CAD build for the part. Positions are in the model's coordinates, mm. Face numbers are marked on the shaded views. Coordinates: 2 decimals unless noted, no trailing zeros. Write each loop counter-clockwise with the first axis right and the second up, starting at its lowest first coordinate (ties: lowest second). Pieces come first, ordered by that corner, then holes. Notation, with made-up numbers: (64.5, -26.75) - (80.5, -26.75) arc R18 cw to (80.5, -7.75) - close; hole circle Ø6 at (-25, 65). An arc over 180 degrees is marked (long way). Answer in a Markdown table with one row per item. Add a question column.
Q1. Band-saw the part on D-D (y = 14). List the corners of the cut face in (x, z).
Q2. Two-plate mould, pull along X, no slides. Class the marked faces 1, 2, 3 and 4: +X half, -X half, draft (parallel to the pull), parting line (faces both ways), or undercut.
Q3. Drill centre lines: line 1 along Y through (x, z) = (-10, -0.25); line 2 along Y through (x, z) = (-13, 2); line 3 along X through (y, z) = (52, 0.4). Where is each one in solid material? Low to high. Write a range as from..to.
Q4. Band-saw the part on B-B (x = -10). List the corners of the cut face in (y, z), and give its area (3 significant figures).
Q5. Band-saw the part on A-A (y = 58). List the corners of the cut face in (x, z).
Q6. Band-saw the part on C-C (z = -0.8). List the corners of the cut face in (x, y), and give its area (3 significant figures).
Autodesk Inventor part; units mm, degrees
ref_plane "YZ Plane" through (0, 0, 0) normal (1, 0, 0) x (0, 1, 0)
ref_plane "XZ Plane" through (0, 0, 0) normal (0, 1, 0) x (-1, 0, 0)
ref_plane "XY Plane" through (0, 0, 0) normal (0, 0, 1) x (1, 0, 0)
sketch "Sketch1" plane through (0, 0, 0) normal (0, 0, 1) x (1, 0, 0)
  line L0 (-5, 0) -> (-15, 0)
  line L1 (-20, 5) -> (-20, 60)
  line L2 (-15, 65) -> (-5, 65)
  line L3 (0, 60) -> (0, 5)
  circle A0 centre (-10, 55) radius 5
  circle A1 centre (-10, 10) radius 5
  arc A2 (-15, 65) -> (-20, 60) centre (-15, 60) ccw
  arc A3 (0, 60) -> (-5, 65) centre (-5, 60) ccw
  arc A4 (-20, 5) -> (-15, 0) centre (-15, 5) ccw
  arc A5 (-5, 0) -> (0, 5) centre (-5, 5) ccw
  point P0 (0, 0)
  point P1 (-20, 65)
  point P2 (-20, 0)
  point P3 (0, 65)
  dimension "d0" = 20
  dimension "d1" = 65
  dimension "d2" = 10
  dimension "d3" = 45
  dimension "d4" = 10
  dimension "d5" = 5
extrude "Extrusion1" add sketch "Sketch1" along normal mid plane 5
sketch "Sketch2" plane through (0, 0, 2.5) normal (0, 0, 1) x (1, 0, 0)
  line L0 (-5, 65) -> (-15, 65)
  arc A0 (-15, 65) -> (-20, 60) centre (-15, 60) ccw
  line L1 (-20, 60) -> (-20, 5)
  arc A1 (-20, 5) -> (-15, 0) centre (-15, 5) ccw
  line L2 (-15, 0) -> (-5, 0)
  arc A2 (-5, 0) -> (0, 5) centre (-5, 5) ccw
  line L3 (0, 5) -> (0, 60)
  arc A3 (0, 60) -> (-5, 65) centre (-5, 60) ccw
  circle A4 centre (-10, 10) radius 5
  circle A5 centre (-10, 55) radius 5
  point P0 (0, 0)
properties part number "Servo arm" material "Aluminum 6061"
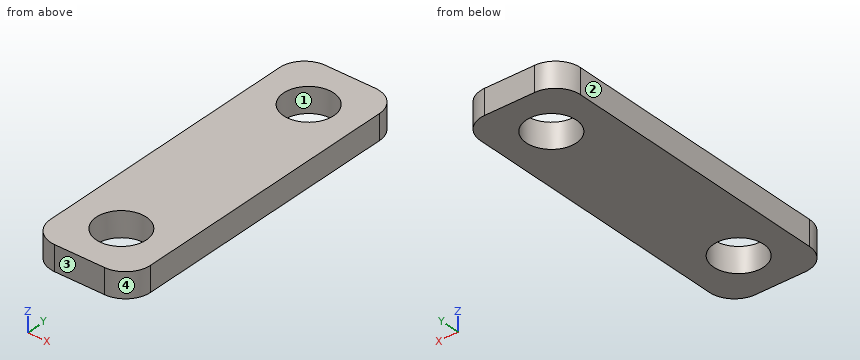
Checked values:
| question | item | result |
|---|---|---|
| 1 | outline | (-20, -2.5) - (-13, -2.5) - (-13, 2.5) - (-20, 2.5) - close; (-7, -2.5) - (0, -2.5) - (0, 2.5) - (-7, 2.5) - close |
| 2 | face 1 | undercut |
| 2 | face 2 | -X half |
| 2 | face 3 | draft |
| 2 | face 4 | +X half |
| 3 | line 1 | y = 0..5, 15..50, 60..65 |
| 3 | line 2 | y = 0..6, 14..51, 59..65 |
| 3 | line 3 | x = -20..-14, -6..0 |
| 4 | outline | (0, -2.5) - (5, -2.5) - (5, 2.5) - (0, 2.5) - close; (15, -2.5) - (50, -2.5) - (50, 2.5) - (15, 2.5) - close; (60, -2.5) - (65, -2.5) - (65, 2.5) - (60, 2.5) - close |
| 4 | area | 225 mm² |
| 5 | outline | (-20, -2.5) - (-14, -2.5) - (-14, 2.5) - (-20, 2.5) - close; (-6, -2.5) - (0, -2.5) - (0, 2.5) - (-6, 2.5) - close |
| 6 | outline | (-20, 5) arc R5 ccw to (-15, 0) - (-5, 0) arc R5 ccw to (0, 5) - (0, 60) arc R5 ccw to (-5, 65) - (-15, 65) arc R5 ccw to (-20, 60) - close; hole circle Ø10 at (-10, 10); hole circle Ø10 at (-10, 55) |
| 6 | area | 1,120 mm² |
